Build history of the part. All positions in model axes, mm. Face numbers are marked on the shaded views. Coordinates: 2 decimals unless noted, no trailing zeros. Order: outer loops, then holes, each group sorted by start corner. A loop starts at its lowest first (then second) coordinate and runs counter-clockwise, first axis right, second up. Notation, with made-up numbers: (20.25, -34) - (41.25, -34) arc R20 cw to (41.25, -1) - close; hole circle Ø3 at (-9.5, -4). An arc over 180 degrees is marked (long way). One line per item, written item: value.
Solid Edge part; units mm, degrees
sketch "Sketch1" plane through (0, 0, 0) normal (0, -1, 0) x (1, 0, 0)
  arc A0 (-100, 50) -> (-400, 50) centre (-250, 50) ccw
  line L0 (-400, -500) -> (-400, 50)
  line L1 (-500, -500) -> (-400, -500)
  line L2 (-500, 500) -> (-500, -500)
  line L3 (500, 500) -> (-500, 500)
  line L4 (500, -500) -> (500, 500)
  line L5 (-100, -500) -> (500, -500)
  line L6 (-100, -500) -> (-100, 50)
extrude "Protrusion1" add sketch "Sketch1" along normal blind 100
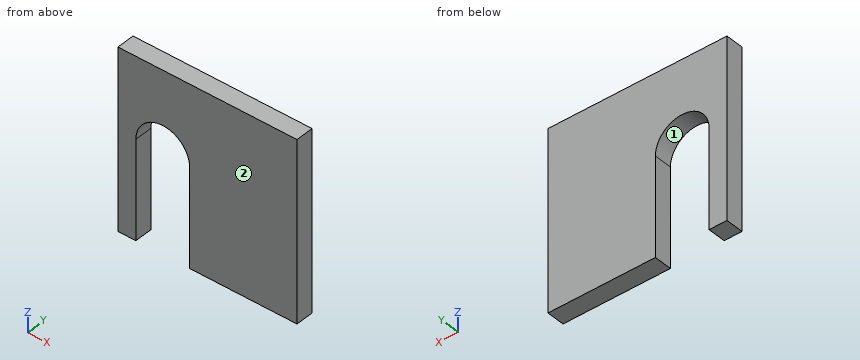
1. Band-saw the part on C-C, the plane x = -250. Give the cut face in (y, z).
Values found:
outline: (-100, 200) - (0, 200) - (0, 500) - (-100, 500) - close
2. Probe line 1 along X through (y, z) = (-13.5, -144.5); line 2 along X through (y, z) = (-34.5, 154.5); line 3 along Z through (x, y) = (-314, -7.5). List the from-to ranges inside material, lowest first.
Values found:
line 1: x = -500 to -400, -100 to 500
line 2: x = -500 to -357.61, -142.39 to 500
line 3: z = 185.66 to 500
3. Band-saw the part on A-A, the plane z = -249.5. Give the cut face in (x, y), and give its area (3 significant figures).
Values found:
outline: (-500, -100) - (-400, -100) - (-400, 0) - (-500, 0) - close; (-100, -100) - (500, -100) - (500, 0) - (-100, 0) - close
area: 70,000 mm2
4. Band-saw the part on D-D, the plane x = -360. Give the cut face in (y, z), and give its area (3 significant figures).
Values found:
outline: (-100, 151.98) - (0, 151.98) - (0, 500) - (-100, 500) - close
area: 34,800 mm2
5. Band-saw the part on B-B, the plane y = -68. Give the cut face in (x, z).
Values found:
outline: (-500, -500) - (-400, -500) - (-400, 50) arc R150 cw to (-100, 50) - (-100, -500) - (500, -500) - (500, 500) - (-500, 500) - close
6. Two-plate mould, pull along X, no slides. Class the marked faces 1 and 2: pulls with the +X half, pulls with the -X half, needs draft (parallel to the pull), parting line crosses it, or undercut.
Values found:
face 1: undercut
face 2: needs draft
7. Flat gauge pin, fed straight in: P1, Ø5, axis at x = -160, y = -43.5, coming from the -Z side. Where does the tip first touch, or does it go through?
Values found:
P1: stops at z = 168.08
